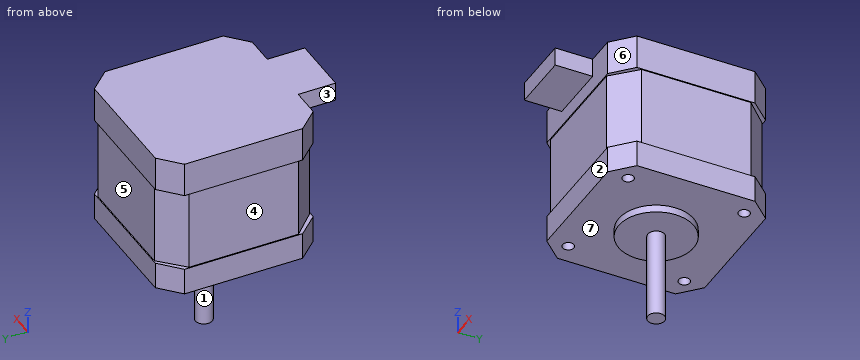
```python
from build123d import *

# Parameters (mm, degrees)
RESSALTO_EXTRUS_O1_DEPTH   = 38
CORTE_EXTRUS_O_FINA1_START = -30.8
CORTE_EXTRUS_O_FINA1_DEPTH = 21.6
ESBO_O3_R                  = 2.25
RESSALTO_EXTRUS_O2_DEPTH   = 26
ESBO_O4_R                  = 10
RESSALTO_EXTRUS_O3_DEPTH   = 2
ESBO_O5_R                  = 1.5
CORTE_EXTRUS_O1_DEPTH      = 10
ESBO_O7_W                  = 16
ESBO_O7_H                  = 5
RESSALTO_EXTRUS_O4_DEPTH   = 10


# Read off the part's stored shape, not the designer's step: Corte-Extrusão-Fina1
with BuildPart() as part:
    # Esboço1 → Ressalto-extrusão1 (new body)
    with BuildSketch(Plane.XY):
        Polygon((-21, -15.592171873), (-15.984175996, -21), (15.592171873, -21), (21, -15.984175996), (21, 15.592171873), (15.984175996, 21), (-15.592171873, 21), (-21, 15.984175996), align=None)
    extrude(amount=RESSALTO_EXTRUS_O1_DEPTH)

    # Corte-Extrusão-Fina1 outline → Corte-Extrusão-Fina1 (cut)
    with BuildSketch(Plane.XY.offset(38).offset(CORTE_EXTRUS_O_FINA1_START)):
        Polygon((15.592171873, -21), (21, -15.984175996), (21, 15.592171873), (15.984175996, 21), (-15.592171873, 21), (-21, 15.984175996), (-21, -15.592171873), (-15.984175996, -21), align=None)
        Polygon((14.605339059, 20.75), (20.75, 14.605339059), (20.75, -14.605339059), (14.605339059, -20.75), (-14.605339059, -20.75), (-20.75, -14.605339059), (-20.75, 14.605339059), (-14.605339059, 20.75), align=None, mode=Mode.SUBTRACT)
    extrude(amount=CORTE_EXTRUS_O_FINA1_DEPTH, mode=Mode.SUBTRACT)

    # Esboço3 → Ressalto-extrusão2 (add)
    with BuildSketch(Plane(origin=(0, 0, 0), x_dir=(-1, 0, 0), z_dir=(0, 0, -1))):
        with Locations(Location((0, 0, 0), (0, 0, 180))):
            Circle(ESBO_O3_R)
    extrude(amount=RESSALTO_EXTRUS_O2_DEPTH)

    # Esboço4 → Ressalto-extrusão3 (add)
    with BuildSketch(Plane(origin=(0, 0, 0), x_dir=(-1, 0, 0), z_dir=(0, 0, -1))):
        with Locations(Location((0, 0, 0), (0, 0, 180))):
            Circle(ESBO_O4_R)
    extrude(amount=RESSALTO_EXTRUS_O3_DEPTH)

    # Esboço5 → Corte-extrusão1 (cut)
    with BuildSketch(Plane(origin=(0, 0, 0), x_dir=(-1, 0, 0), z_dir=(0, 0, -1))):
        with Locations((15.5, -15.5)):
            Circle(ESBO_O5_R)
        with Locations((-15.5, -15.5)):
            Circle(ESBO_O5_R)
        with Locations((-15.5, 15.5)):
            Circle(ESBO_O5_R)
        with Locations((15.5, 15.5)):
            Circle(ESBO_O5_R)
    extrude(amount=-CORTE_EXTRUS_O1_DEPTH, mode=Mode.SUBTRACT)

    # Esboço7 → Ressalto-extrusão4 (add)
    with BuildSketch(Plane.XZ.offset(21)):
        with Locations((-0.196002062, 35.5)):
            Rectangle(ESBO_O7_W, ESBO_O7_H)
    extrude(amount=RESSALTO_EXTRUS_O4_DEPTH)


solid = part.part
```
Check sheet for the modelled part. Datum: model origin and axes. Units: mm. Face numbers are marked on the shaded views. A direction names the side the tool comes from. Give positions to 0.01 mm unless a question says otherwise; leave off trailing zeros. Write each loop counter-clockwise with the first axis right and the second up, starting at its lowest first coordinate (ties: lowest second). Pieces come first, ordered by that corner, then holes.
Item 1: Gauge pin test, flat ends, axial feed: pin 1 (8 mm diameter, centred on x = -3, y = -24, fed in from -Z); pin 2 (1.5 mm diameter, centred on y = -26.5, z = 36, fed in from +X); pin 3 (1.5 mm diameter, centred on y = 2.5, z = -15.5, fed in from +X). Record the tip position at first contact, or that the pin passes through.
Item 2: Cross-section at B-B (y = 0). Enter the section's corners in (x, z), and give its area (3 significant figures).
Item 3: Cross-section at C-C (z = -7.5). Enter the section's corners in (x, y).
Item 4: Scan lines: L1, parallel to Y at x = -15.5, z = 5; L2, parallel to Y at x = 15, z = 7. Record each from-to range of solid material in increasing order.
Item 5: Cross-section at D-D (x = 6.5). Enter the section's corners in (y, z), and give its area (3 significant figures).
Item 6: Cross-section at A-A (x = -11). Enter the section's corners in (y, z).
Item 7: Access from +Z, -Z, +X, -X, +Y, -Y to the whole of each face (thin tool, end or side, straight path). Record for the marked faces 1, 2, 3 and 4.
Item 8: Draft check along Z on the marked faces 5, 6 and 7. Enter one of: released by +Z, released by -Z, zero draft, split by the parting line, or undercut.
Report:
1. pin 1: stops at z = 0
1. pin 2: stops at x = 7.8
1. pin 3: stops at x = 1.41
2. outline: (-21, 0) - (-10, 0) - (-10, -2) - (-2.25, -2) - (-2.25, -26) - (2.25, -26) - (2.25, -2) - (10, -2) - (10, 0) - (21, 0) - (21, 7.2) - (20.75, 7.2) - (20.75, 28.8) - (21, 28.8) - (21, 38) - (-21, 38) - (-21, 28.8) - (-20.75, 28.8) - (-20.75, 7.2) - (-21, 7.2) - close
2. area: 1,730 mm2
3. outline: circle Ø4.5 at (0, 0)
4. L1: y = -21 to -17, -14 to 14, 17 to 21
4. L2: y = -21 to -16.91, -14.09 to 14.09, 16.91 to 21
5. outline: (-31, 33) - (-21, 33) - (-21, 28.8) - (-20.75, 28.8) - (-20.75, 7.2) - (-21, 7.2) - (-21, 0) - (-7.6, 0) - (-7.6, -2) - (7.6, -2) - (7.6, 0) - (21, 0) - (21, 7.2) - (20.75, 7.2) - (20.75, 28.8) - (21, 28.8) - (21, 38) - (-31, 38) - close
5. area: 1,670 mm2
6. outline: (-21, 0) - (21, 0) - (21, 7.2) - (20.75, 7.2) - (20.75, 28.8) - (21, 28.8) - (21, 38) - (-21, 38) - (-21, 28.8) - (-20.75, 28.8) - (-20.75, 7.2) - (-21, 7.2) - close
7. face 1: -Z
7. face 2: -Z, +X, -X, -Y
7. face 3: +Z, -Z, -X, -Y
7. face 4: -X, +Y, -Y
8. face 5: undercut
8. face 6: zero draft
8. face 7: released by -Z
